Source: CAD feature listing. Evaluate the final solid. Frame: model axes, mm. A direction names the side the tool comes from. Give positions to 0.01 mm unless a question says otherwise; leave off trailing zeros. Write each loop counter-clockwise with the first axis right and the second up, starting at its lowest first coordinate (ties: lowest second). Pieces come first, ordered by that corner, then holes. Notation, with made-up numbers: M -29,89.5 L 25,89.5 A31 ccw 25,121.5 Z; hole C 70.25,-33.5 d5. An arc over 180 degrees is marked long. Return JSON: item names as keys, results as strings.
```python
from build123d import *

# Parameters (mm, degrees)
ESQUISSE1_R        = 7
ESQUISSE1_R_2      = 4
BOSS_EXTRU_1_DEPTH = 25
CHANFREIN1_SIZE    = 0.25
BOSS_EXTRU_2_START = 5
ESQUISSE2_R        = 1.5
BOSS_EXTRU_2_DEPTH = 3


with BuildPart() as part:
    # Esquisse1 → Boss.-Extru.1 (new body)
    with BuildSketch(Plane.XY):
        Circle(ESQUISSE1_R)
        Circle(ESQUISSE1_R_2, mode=Mode.SUBTRACT)
    extrude(amount=BOSS_EXTRU_1_DEPTH)

    # Chanfrein1
    chanfrein1_edges = [part.edges().sort_by_distance(p)[0] for p in [
        (-7, 0, 0),
        (-7, 0, 25),
        (-4, 0, 0),
        (-4, 0, 25),
    ]]
    chamfer(chanfrein1_edges, length=CHANFREIN1_SIZE)

    # Esquisse2 → Boss.-Extru.2 (add)
    with BuildSketch(Plane(origin=(0, 0, 0), x_dir=(1, 0, 0), z_dir=(0, 1, 0)).offset(BOSS_EXTRU_2_START)):
        with Locations(Location((0, -4.25, 0), (0, 0, 90))):
            Circle(ESQUISSE2_R)
        with Locations(Location((0, -20.75, 0), (0, 0, 90))):
            Circle(ESQUISSE2_R)
    extrude(amount=BOSS_EXTRU_2_DEPTH)


solid = part.part
```
1) Contact query for flat-ended pins moving along their axis: pin 1 Ø3 at (x, z) = (5.5, 16.5) entering from -Y; pin 2 Ø3 at (y, z) = (4, 16.5) entering from -X; pin 3 Ø1.5 at (x, z) = (1, 15) entering from +Y. Output: stop coordinate, or through.
Numbers:
{"pin 1": "stops at y = -5.74", "pin 2": "stops at x = -6.54", "pin 3": "stops at y = 7"}
2) Draft query along X for faces 3 (the face through (-0.45, 7.41, 19.32)), 4 (the face through (0, 8, 4)), 5 (the face through (-0.867, -3.905, 12.328)). Return one class per face: released by +X, released by -X, zero draft, split by the parting line, or undercut.
Numbers:
{"face 3": "split by the parting line", "face 4": "zero draft", "face 5": "undercut"}
3) Cut plane C-C, the plane z = 15.75. Return the cut outline in (x, y).
Numbers:
{"outline": "C 0,0 d14; hole C 0,0 d8"}
4) Cut plane A-A, the plane x = 0. Return the cut outline in (y, z), then the cut area to 3 significant figures.
Numbers:
{"outline": "M -7,0.25 L -6.75,0 L -4.25,0 L -4,0.25 L -4,24.75 L -4.25,25 L -6.75,25 L -7,24.75 Z; M 4,0.25 L 4.25,0 L 6.75,0 L 7,0.25 L 7,2.75 L 8,2.75 L 8,5.75 L 7,5.75 L 7,19.25 L 8,19.25 L 8,22.25 L 7,22.25 L 7,24.75 L 6.75,25 L 4.25,25 L 4,24.75 Z", "area": "156 mm²"}
5) Line query: line 1 (Y direction, x = 0, z = 18); line 2 (X direction, y = 1.5, z = 4.25); line 3 (X direction, y = 0.25, z = 3.5). Output: solid intervals per line, ascending. Write a range as [from, to].
Numbers:
{"line 1": "y = [-7, -4], [4, 7]", "line 2": "x = [-6.84, -3.71], [3.71, 6.84]", "line 3": "x = [-7, -3.99], [3.99, 7]"}
6) Cut plane B-B, the plane z = 4.25. Return the cut outline in (x, y), then the cut area to 3 significant figures.
Numbers:
{"outline": "M -1.5,6.84 A7 ccw long 1.5,6.84 L 1.5,8 L -1.5,8 Z; hole C 0,0 d8", "area": "107 mm²"}
7) Set-up query: faces 1 (the face through (4.4, 0.1, 0)), 2 (the face through (-0.45, 7.41, 2.82)). Return all of +Z, -Z, +X, -X, +Y, -Y with unobstructed straight access to the full face (end or side cutting, diameter ignored); none if empty.
Numbers:
{"face 1": "-Z, +X, -X, +Y, -Y", "face 2": "+Y"}
